from build123d import *

# Parameters (mm, degrees)
SKETCH1_W           = 1180
SKETCH1_H           = 150
BOSS_EXTRUDE1_DEPTH = 120
SKETCH2_R           = 50
CUT_EXTRUDE1_DEPTH  = 50
CHAMFER1_SIZE       = 210
CHAMFER1_SIZE2      = 97.924608213
SKETCH3_W           = 170
SKETCH3_H           = 102
CUT_EXTRUDE2_DEPTH  = 10
FILLET2_R           = 10
SKETCH4_W           = 170
SKETCH4_H           = 102
CUT_EXTRUDE3_DEPTH  = 10
FILLET3_R           = 10
FILLET4_R           = 10


with BuildPart() as part:
    # Sketch1 → Boss-Extrude1 (new body)
    with BuildSketch(Plane(origin=(0, 0, 0), x_dir=(1, 0, 0), z_dir=(0, 1, 0))):
        with Locations((0, -75)):
            Rectangle(SKETCH1_W, SKETCH1_H)
    extrude(amount=-BOSS_EXTRUDE1_DEPTH)

    # Sketch2 → Cut-Extrude1 (cut)
    with BuildSketch(Plane(origin=(0, 0, 0), x_dir=(-1, 0, 0), z_dir=(0, 0, -1))):
        with Locations((-515, -60)):
            Circle(SKETCH2_R)
        with Locations((515, -60)):
            Circle(SKETCH2_R)
    extrude(amount=-CUT_EXTRUDE1_DEPTH, mode=Mode.SUBTRACT)

    # Chamfer1
    chamfer1_edges = [part.edges().sort_by_distance(p)[0] for p in [
        (590, -60, 150),
        (-590, -60, 150),
    ]]
    chamfer1_side = [part.faces().sort_by_distance(p)[0] for p in [
        (0, -60, 150),
    ]]
    chamfer(chamfer1_edges, length=CHAMFER1_SIZE, length2=CHAMFER1_SIZE2, reference=chamfer1_side[0])

    # Sketch3 → Cut-Extrude2 (cut)
    with BuildSketch(Plane(origin=(-125.323687393, 0, 268.757514919), x_dir=(0.9063077870366509, 0, 0.42261826174069755), z_dir=(-0.4226182617406975, 0, 0.9063077870366508))):
        with Locations((-398.858582795, -60)):
            Rectangle(SKETCH3_W, SKETCH3_H)
    cut_extrude2 = extrude(amount=-CUT_EXTRUDE2_DEPTH, mode=Mode.SUBTRACT)

    # Fillet2
    fillet2_edges = [part.edges().sort_by_distance(p)[0] for p in [
        (-561.735397496, -111, 59.738502795),
        (-561.735397496, -9, 59.738502795),
        (-407.6630737, -9, 131.583607291),
        (-407.6630737, -111, 131.583607291),
    ]]
    fillet(fillet2_edges, radius=FILLET2_R)

    # Mirror1: Cut-Extrude2 across plane
    add(cut_extrude2.mirror(Plane(origin=(0, 0, 0), x_dir=(0, 0, 1), z_dir=(1, 0, 0))), mode=Mode.SUBTRACT)

    # Sketch4 → Cut-Extrude3 (cut)
    with BuildSketch(Plane.XY.offset(150)):
        with Locations((-245, -60)):
            Rectangle(SKETCH4_W, SKETCH4_H)
    cut_extrude3 = extrude(amount=-CUT_EXTRUDE3_DEPTH, mode=Mode.SUBTRACT)

    # Fillet3
    fillet3_edges = [part.edges().sort_by_distance(p)[0] for p in [
        (-330, -111, 145),
        (-330, -9, 145),
        (-160, -9, 145),
        (-160, -111, 145),
    ]]
    fillet(fillet3_edges, radius=FILLET3_R)

    # Mirror2: Cut-Extrude3 across plane
    add(cut_extrude3.mirror(Plane(origin=(0, 0, 0), x_dir=(0, 0, 1), z_dir=(1, 0, 0))), mode=Mode.SUBTRACT)

    # Fillet4
    fillet4_edges = [part.edges().sort_by_distance(p)[0] for p in [
        (330, -9, 145),
        (330, -111, 145),
        (160, -111, 145),
        (160, -9, 145),
        (561.735397496, -9, 59.738502795),
        (561.735397496, -111, 59.738502795),
        (407.6630737, -111, 131.583607291),
        (407.6630737, -9, 131.583607291),
    ]]
    fillet(fillet4_edges, radius=FILLET4_R)


solid = part.part
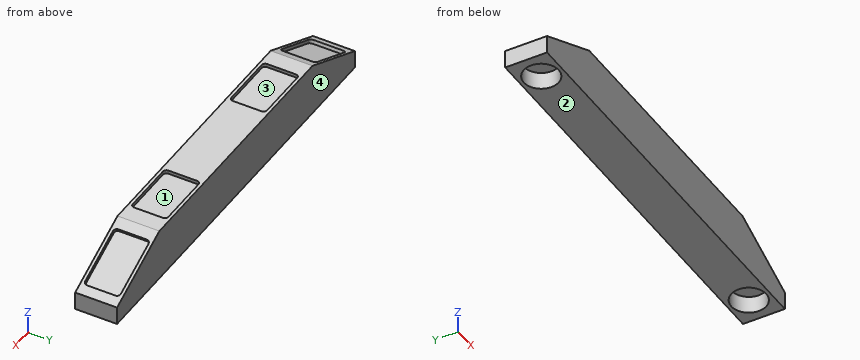
Build history of the part. All positions in model axes, mm. Face numbers are marked on the shaded views. A direction names the side the tool comes from. Coordinates: 2 decimals unless noted, no trailing zeros. Write each loop counter-clockwise with the first axis right and the second up, starting at its lowest first coordinate (ties: lowest second). Pieces come first, ordered by that corner, then holes.
(1) Drill centre lines: line 1 (X direction, y = -90, z = 14.5); line 2 (Y direction, x = 515, z = 15); line 3 (X direction, y = -96, z = 44). Where is each one in solid material? Low to high.
(2) Pin check, flat tips, straight feed: pin 1 Ø4 at (y, z) = (-60, 59.5) entering from +X; pin 2 Ø3 at (y, z) = (-49.5, 146) entering from -X; pin 3 Ø4 at (y, z) = (-43, 75.5) entering from +X. Stop position of each tip, or through.
(3) Cut at C-C on z = 111. List the corners of the cut face in (x, y).
(4) Cut at B-B on x = -271.5. List the corners of the cut face in (y, z), and give its area (3 significant figures).
(5) Cut at D-D on x = 515. List the corners of the cut face in (y, z), and give its area (3 significant figures).
(6) Mould opens along X. For the marked faces 3 and 4 say: pulls with the +X half, pulls with the -X half, needs draft (parallel to the pull), parting line crosses it, or undercut.
(7) 3-axis set-ups, long thin cutter, end or side, ignore diameter. For the marked faces 1 and 2: which of +Z, -Z, +X, -X, +Y, -Y reach the whole face in a straight line?
Working result:
1. line 1: x = -590 to -555, -475 to 475, 555 to 590
1. line 2: y = -120 to -110, -10 to 0
1. line 3: x = -590 to -549.7, -480.3 to 480.3, 549.7 to 590
2. pin 1: stops at x = 578.37
2. pin 2: stops at x = -391.79
2. pin 3: stops at x = 520.39
3. outline: (-463.64, -120) - (463.64, -120) - (463.64, -111) - (439.97, -111) - (439.97, -9) - (463.64, -9) - (463.64, 0) - (-463.64, 0) - (-463.64, -9) - (-439.97, -9) - (-439.97, -111) - (-463.64, -111) - close
4. outline: (-120, 0) - (0, 0) - (0, 150) - (-9, 150) - (-9, 140) - (-111, 140) - (-111, 150) - (-120, 150) - close
4. area: 17,000 mm2
5. outline: (-120, 0) - (-110, 0) - (-110, 50) - (-10, 50) - (-10, 0) - (0, 0) - (0, 87.05) - (-9, 87.05) - (-9, 76.01) - (-111, 76.01) - (-111, 87.05) - (-120, 87.05) - close
5. area: 4,320 mm2
6. face 3: undercut
6. face 4: needs draft
7. face 1: +Z
7. face 2: -Z, +X, -X, +Y, -Y
